Check sheet for the modelled part. Datum: model origin and axes. Units: mm. Face numbers are marked on the shaded views. A direction names the side the tool comes from. Round coordinates to 2 decimals unless told otherwise and drop trailing zeros. Loops run counter-clockwise (first coordinate to the right, second up) from the corner with the lowest first, then second, coordinate; pieces in that order, holes last. Notation, with made-up numbers: (87.5, -1.75) -> (135.5, -1.75) arc R4 cw to (135.5, 5.25) -> close; hole circle Ø5 at (25.25, -28.75). An arc over 180 degrees is marked (long way). One line per question, with ' | ' between items.
```python
from build123d import *

# Parameters (mm, degrees)
SZKIC2_R                   = 3.25
SZKIC2_R_2                 = 1.1
SZKIC2_W                   = 5
SZKIC2_H                   = 41.231056256
WYTNIJ_WYCI_GNI_CIE1_DEPTH = 76.166481892


with BuildPart() as part:
    # Szkic1 → Obrót1 (revolve)
    with BuildSketch(Plane.XY, mode=Mode.PRIVATE) as obr_t1_sk:
        Polygon((-2, 9.5), (-2, 20), (-40, 20), (-40, 45), (-35, 45), (-35, 22.5), (0, 22.5), (0, 9.5), align=None)
    revolve(obr_t1_sk.sketch.rotate(Axis((0, 0, 0), (-1, 0, 0)), 90), axis=Axis((0, 0, 0), (-1, 0, 0)))

    # Szkic2 → Wytnij-wyciągnięcie1 (cut, through all)
    with BuildSketch(Plane(origin=(0, 0, 0), x_dir=(0, 0, -1), z_dir=(1, 0, 0))):
        with Locations((26.516504294, 26.516504294)):
            Circle(SZKIC2_R)
        with Locations((26.516504294, -26.516504294)):
            Circle(SZKIC2_R)
        with Locations((-26.516504294, -26.516504294)):
            Circle(SZKIC2_R)
        with Locations((-26.516504294, 26.516504294)):
            Circle(SZKIC2_R)
        with Locations((0, 11.25)):
            Circle(SZKIC2_R_2)
        with Locations((9.742785793, 5.625)):
            Circle(SZKIC2_R_2)
        with Locations((9.742785793, -5.625)):
            Circle(SZKIC2_R_2)
        with Locations((0, -11.25)):
            Circle(SZKIC2_R_2)
        with Locations((-9.742785793, -5.625)):
            Circle(SZKIC2_R_2)
        with Locations((-9.742785793, 5.625)):
            Circle(SZKIC2_R_2)
        with Locations((-42.5, 0)):
            Rectangle(SZKIC2_W, SZKIC2_H)
        with Locations((42.5, 0)):
            Rectangle(SZKIC2_W, SZKIC2_H)
    extrude(amount=-WYTNIJ_WYCI_GNI_CIE1_DEPTH, mode=Mode.SUBTRACT)


solid = part.part
```
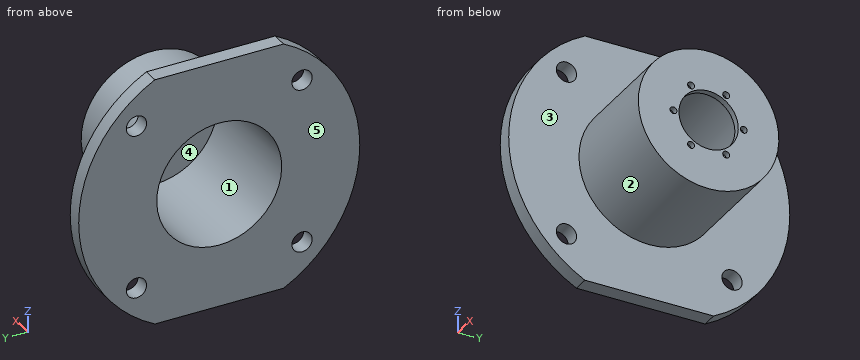
(1) Scan lines: probe 1 along Y at (x, z) = (-15.5, 0); probe 2 along X at (y, z) = (6, -32); probe 3 along X at (y, z) = (7, 17). Record each from-to range of solid material in increasing order.
Answer:
probe 1: y = -22.5 to -20, 20 to 22.5 | probe 2: x = -40 to -35 | probe 3: x = -2 to 0
(2) Sectioned sample at B-B, the plane z = -6. Record the cut outline in (x, y).
Answer:
outline: (-40, -44.6) -> (-35, -44.6) -> (-35, -21.69) -> (0, -21.69) -> (0, -7.37) -> (-2, -7.37) -> (-2, -19.08) -> (-40, -19.08) -> close; (-40, 19.08) -> (-2, 19.08) -> (-2, 7.37) -> (0, 7.37) -> (0, 21.69) -> (-35, 21.69) -> (-35, 44.6) -> (-40, 44.6) -> close
(3) Sectioned sample at A-A, the plane y = 0. Record the cut outline in (x, z), and give its area (3 significant figures).
Answer:
outline: (-40, -40) -> (-35, -40) -> (-35, -22.5) -> (0, -22.5) -> (0, -9.5) -> (-2, -9.5) -> (-2, -20) -> (-40, -20) -> close; (-40, 20) -> (-2, 20) -> (-2, 9.5) -> (0, 9.5) -> (0, 22.5) -> (-35, 22.5) -> (-35, 40) -> (-40, 40) -> close | area: 417 mm2
(4) Mould release check, pull along Y, two halves, no side actions. Record for the marked faces 1, 2 and 3: +Y half, -Y half, draft (parallel to the pull), parting line (faces both ways), or undercut.
Answer:
face 1: undercut | face 2: parting line | face 3: draft
(5) Go/stop test with flat-tipped pins: pin 1 (3.5 mm diameter, centred on y = 11.25, z = 0, fed in from -X); pin 2 (5 mm diameter, centred on y = -26.52, z = 26.52, fed in from -X); pin 3 (8.5 mm diameter, centred on y = -26.52, z = -26.52, fed in from +X); pin 4 (4 mm diameter, centred on x = -20.5, y = -20.5, fed in from -Z). Record where each tip stops, or that it passes through.
Answer:
pin 1: stops at x = -2 | pin 2: passes through | pin 3: stops at x = -35 | pin 4: stops at z = -12.81
(6) Sectioned sample at D-D, the plane x = -31. Record the cut outline in (y, z), and give its area (3 significant figures).
Answer:
outline: circle Ø45 at (0, 0); hole circle Ø40 at (0, 0) | area: 334 mm2
(7) Sectioned sample at C-C, the plane z = -28. Record the cut outline in (x, y).
Answer:
outline: (-40, -35.23) -> (-35, -35.23) -> (-35, -29.41) -> (-40, -29.41) -> close; (-40, -23.62) -> (-35, -23.62) -> (-35, 23.62) -> (-40, 23.62) -> close; (-40, 29.41) -> (-35, 29.41) -> (-35, 35.23) -> (-40, 35.23) -> close
(8) Set-up check for the marked faces 4 and 5: record each of +Z, -Z, +X, -X, +Y, -Y from which the full face is reachable in a straight line by a thin tool's end or side.
Answer:
face 4: -X | face 5: +Z, -Z, -X, +Y, -Y
